Geometry: final body of the model. Coordinates: model frame, mm. A direction names the side the tool comes from. Give positions to 0.01 mm unless a question says otherwise; leave off trailing zeros. Write each loop counter-clockwise with the first axis right and the second up, starting at its lowest first coordinate (ties: lowest second). Pieces come first, ordered by that corner, then holes.
Q1. Pin query (flat end, axial travel): pin 1 (3 mm diameter, centred on x = 2.5, y = 4, fed in from +Z); pin 2 (1.2 mm diameter, centred on y = 4.5, z = -0.5, fed in from +X); pin 3 (1.3 mm diameter, centred on x = 8.5, y = 3, fed in from -Z). Return the tip coordinate at first contact, or that it passes through.
Q2. Cut plane C-C on x = 0. Return the cut outline in (y, z).
Q3. Cut plane B-B on z = 0. Return the cut outline in (x, y).
Q4. Draft query along X for faces 1 (the face through (-2.3, 2, 2.3)), 2 (the face through (8, 3, 3)), 3 (the face through (-7, 3, 7)). Return one class per face: pulls with the +X half, pulls with the -X half, needs draft (parallel to the pull), parting line crosses it, or undercut.
Q5. Cut plane A-A on y = 3.1. Return the cut outline in (x, z), plus the area to 3 significant figures.
Q6. Cut plane D-D on y = 0.7. Return the cut outline in (x, z), plus the area to 3 significant figures.
Q7. Reachability of faces 4 (the face through (7, 3, -7)), 5 (the face through (8, 3, -3)), 6 (the face through (0, 3, -6.9)), 7 (the face through (5, 4, 0)) from +Z, -Z, +X, -X, +Y, -Y: full face, straight path, thin tool, end or side. Return the list, or none.
Q8. Line query: L1, parallel to X at y = 0.6, z = 0; L2, parallel to Z at x = 0.25, y = 3.4; L3, parallel to X at y = 3.75, z = 0. Output: solid intervals per line, ascending.
```python
from build123d import *

# Parameters (mm, degrees)
SKETCH1_W           = 10
SKETCH1_H           = 10
BOSS_EXTRUDE1_DEPTH = 6
SKETCH3_W           = 10
SKETCH3_H           = 10
SKETCH3_R           = 3.1
BOSS_EXTRUDE2_DEPTH = 2


with BuildPart() as part:
    # Sketch1 → Boss-Extrude1 (new body)
    with BuildSketch(Plane(origin=(0, 0, 0), x_dir=(1, 0, 0), z_dir=(0, 1, 0))):
        with BuildLine():
            Line((6.9, -3), (6.9, 3))
            Line((6.9, 3), (9.434511116, 3))
            ThreePointArc((9.434511116, 3), (7.000357134, 7.000357134), (3, 9.434511116))
            Line((3, 9.434511116), (3, 6.9))
            Line((3, 6.9), (-3, 6.9))
            Line((-3, 6.9), (-3, 9.434511116))
            ThreePointArc((-3, 9.434511116), (-7.000357134, -7.000357134), (9.434511116, -3))
            Line((9.434511116, -3), (6.9, -3))
        make_face()
        Rectangle(SKETCH1_W, SKETCH1_H, mode=Mode.SUBTRACT)
    extrude(amount=BOSS_EXTRUDE1_DEPTH)

    # Sketch3 → Boss-Extrude2 (add)
    with BuildSketch(Plane.XZ):
        Rectangle(SKETCH3_W, SKETCH3_H)
        with Locations(Location((0, 0, 0), (0, 0, 270))):
            Circle(SKETCH3_R, mode=Mode.SUBTRACT)
    extrude(amount=-BOSS_EXTRUDE2_DEPTH)


solid = part.part
```
Data:
1. pin 1: stops at z = 9.85
1. pin 2: stops at x = 6.9
1. pin 3: stops at z = -6.03
2. outline: (0, -6.9) - (6, -6.9) - (6, -5) - (2, -5) - (2, -3.1) - (0, -3.1) - close; (0, 3.1) - (2, 3.1) - (2, 5) - (6, 5) - (6, 9.9) - (0, 9.9) - close
3. outline: (-9.9, 0) - (-3.1, 0) - (-3.1, 2) - (-5, 2) - (-5, 6) - (-9.9, 6) - close; (3.1, 0) - (6.9, 0) - (6.9, 6) - (5, 6) - (5, 2) - (3.1, 2) - close
4. face 1: undercut
4. face 2: needs draft
4. face 3: parting line crosses it
5. outline: (-3, -9.43) - (-3, -6.9) - (3, -6.9) - (3, -9.43) arc R9.9 ccw to (9.43, -3) - (6.9, -3) - (6.9, 3) - (9.43, 3) arc R9.9 ccw (long way) to start; hole (-5, -5) - (5, -5) - (5, 5) - (-5, 5) - close
5. area: 174 mm2
6. outline: (-3, -9.43) - (-3, -6.9) - (3, -6.9) - (3, -9.43) arc R9.9 ccw to (9.43, -3) - (6.9, -3) - (6.9, 3) - (9.43, 3) arc R9.9 ccw (long way) to start; hole circle Ø6.2 at (0, 0)
6. area: 244 mm2
7. face 4: -Z, +X, +Y, -Y
7. face 5: +X, +Y, -Y
7. face 6: -Z, +Y, -Y
7. face 7: +Y
8. L1: x = -9.9 to -3.1, 3.1 to 6.9
8. L2: z = -6.9 to -5, 5 to 9.9
8. L3: x = -9.9 to -5, 5 to 6.9
